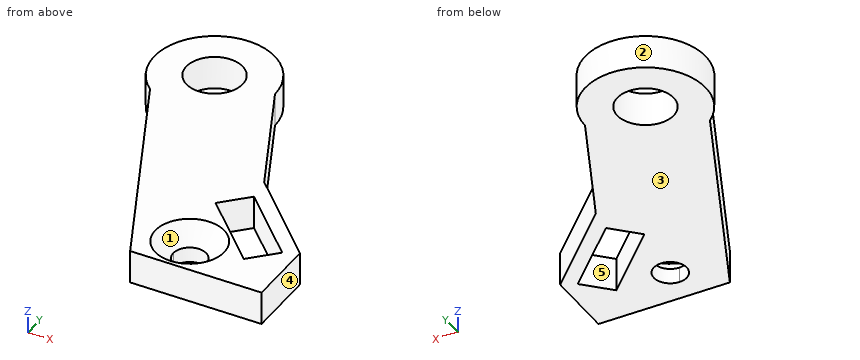
```python
from build123d import *

# Parameters (mm, degrees)
SKETCH1_R           = 2.575
BOSS_EXTRUDE1_DEPTH = 3.05


with BuildPart() as part:
    # Sketch1 → Boss-Extrude1 (new body)
    with BuildSketch(Plane.XY):
        with BuildLine():
            Line((0, 0), (12, 0))
            Line((12, 0), (12, 6.303908615))
            Line((12, 6.303908615), (4.681585686, 13.62232293))
            Line((4.681585686, 13.62232293), (-0.534038586, 24.807265275))
            ThreePointArc((-0.534038586, 24.807265275), (-8.358318048, 29.755478813), (-9.597116456, 20.581082657))
            Line((-9.597116456, 20.581082657), (0, 0))
        make_face()
        Polygon((10.727207794, 5.692209589), (8.464466094, 3.429467889), (2.701545827, 9.192388155), (4.964287527, 11.455129855), align=None, mode=Mode.SUBTRACT)
        with BuildLine():
            ThreePointArc((2, 3.5), (4.560660172, 4.560660172), (3.5, 2))
            Line((3.5, 2), (3.5, 3.5))
            Line((3.5, 3.5), (2, 3.5))
        make_face(mode=Mode.SUBTRACT)
        with Locations((-6.033917608, 24.770785985)):
            Circle(SKETCH1_R, mode=Mode.SUBTRACT)
    extrude(amount=BOSS_EXTRUDE1_DEPTH)

    # Sketch3 → CSK for M3 Flat Head Machine Screw1 (revolve, cut)
    with BuildSketch(Plane(origin=(3.5, 3.5, 3.05), x_dir=(0, -1, 0), z_dir=(1, 0, 0))):
        Polygon((0, 0), (0, 3.05), (1.5, 3.05), (1.5, 1.65), (3.15, 0), align=None)
    revolve(axis=Axis((3.5, 3.5, 9.4), (0, 0, -1)), mode=Mode.SUBTRACT)


solid = part.part
```
Can you work these out from the model? Positions are in its coordinate system, mm. Face numbers are marked on the shaded views. A direction names the side the tool comes from. Give positions to 0.01 mm unless a question says otherwise; leave off trailing zeros. Loops run counter-clockwise (first coordinate to the right, second up) from the corner with the lowest first, then second, coordinate; pieces in that order, holes last. Notation, with made-up numbers: M 30,45 L 74,45 A12 ccw 74,56 Z; hole C 89,-19.75 d1. An arc over 180 degrees is marked long. Use one line per item in the form item = value. Start each with the question number.
(1) Please list where these lines run through material, in increasing order: line 1 (Y direction, x = 3.5, z = 1.05); line 2 (Y direction, x = 3.5, z = 2.4); line 3 (X direction, y = 25.5, z = 0.25).
(2) I want a section at B-B, the plane x = 9.25. Write out the boundary of the cut face in (y, z) (3 decimals), and give its area (3 significant figures).
(3) I'm going to push a flat-ended pin straight in: P1, Ø1.5, axis at x = -1.5, z = 1, coming from the -Y side. Where does the tip first touch, or does it pass through?
(4) I want a section at A-A, the plane y = 7.5. Write out the boundary of the cut face in (x, z).
(5) On a 3-axis mill with a long thin cutter (end or side, diameter ignored), from which of +Z, -Z, +X, -X, +Y, -Y can I reach the whole of each face in a straight line? I mean the marked faces 4 and 5. Say none if no direction works.
(6) I want a section at C-C, the plane z = 1.9. Write out the boundary of the cut face in (x, y) (3 decimals).
(7) Thinking about a two-plate mould opening in Z: for the marked faces 1, 2 and 3, which applies, released by +Z, released by -Z, zero draft, split by the parting line, or undercut?
Worked out:
q1.line_1 = 0 to 2, 5 to 8.39, 9.99 to 16.16
q1.line_2 = 0 to 1, 6 to 8.39, 9.99 to 16.16
q1.line_3 = -11.49 to -8.5, -3.56 to -0.58
q2.outline = M 0,0 L 4.215,0 L 4.215,3.05 L 0,3.05 Z; M 7.169,0 L 9.054,0 L 9.054,3.05 L 7.169,3.05 Z
q2.area = 18.6 mm²
q3.P1 = 1.61
q4.outline = M -3.5,0 L 4.39,0 L 4.39,3.05 L -3.5,3.05 Z; M 8.92,0 L 10.8,0 L 10.8,3.05 L 8.92,3.05 Z
q5.face_4 = +Z, -Z, +X, +Y, -Y
q5.face_5 = +Z, -Z
q6.outline = M -9.597,20.581 L 0,0 L 12,0 L 12,6.304 L 4.682,13.622 L -0.534,24.807 A5.5 ccw long Z; hole C -6.034,24.771 d5.15; hole C 3.5,3.5 d4; hole M 2.702,9.192 L 8.464,3.429 L 10.727,5.692 L 4.964,11.455 Z
q7.face_1 = released by +Z
q7.face_2 = zero draft
q7.face_3 = released by -Z
